Could you check a few things on this model? Use its own coordinates, in mm. Give positions to 0.01 mm unless a question says otherwise; leave off trailing zeros. Order: outer loops, then holes, each group sorted by start corner. A loop starts at its lowest first (then second) coordinate and runs counter-clockwise, first axis right, second up. Notation, with made-up numbers: (-15, -9.75) -> (19, -9.75) arc R17 ccw to (19, 9.25) -> close; hole circle Ø7 at (9.5, 7.5). An arc over 180 degrees is marked (long way). One line per item, written item: value.
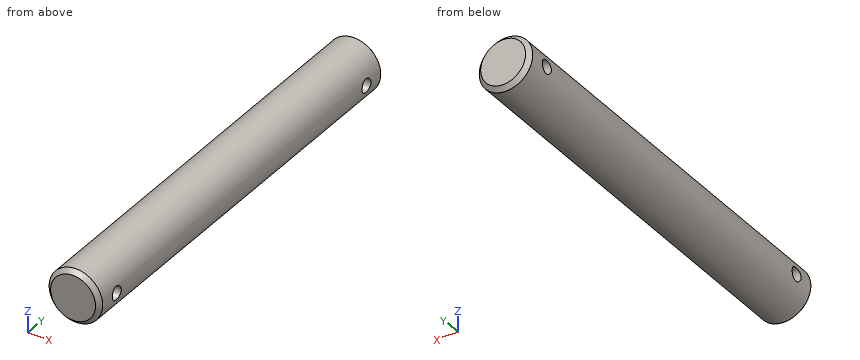
```python
from build123d import *

# Parameters (mm, degrees)
F0_R     = 12.5
F1_DEPTH = 200
F2_R     = 3.15
F3_DEPTH = 65
F4_SIZE  = 2


with BuildPart() as f1:
    # F0 (on Front) → F1 (new body)
    with BuildSketch(Plane.XZ):
        Circle(F0_R)
    extrude(amount=F1_DEPTH)

    # F2 (on Right) → F3 (cut, symmetric)
    with BuildSketch(Plane.YZ):
        with Locations((-12, 0)):
            Circle(F2_R)
        with Locations((-188, 0)):
            Circle(F2_R)
    extrude(amount=F3_DEPTH, both=True, mode=Mode.SUBTRACT)

    # F4
    f4_edges = [f1.edges().sort_by_distance(p)[0] for p in [
        (-12.5, 0, 0),
        (-12.5, -200, 0),
    ]]
    chamfer(f4_edges, length=F4_SIZE)


solid = f1.part
```
1) Suppose I cut it at C-C, the plane y = -90.5. Write out the boundary of the cut face in (x, z).
Answer below:
outline: circle Ø25 at (0, 0)
2) For P1, Ø10, axis at x = 5, y = -38, coming from the +Z side; P2, Ø4, axis at y = -46.5, z = -5.5, coming from the +X side; P3, Ø4, axis at y = -88.5, z = -8, coming from the -X side, each with a flat end and sliding along its axis, tell me the tip position at first contact or that it passes through.
Answer below:
P1: stops at z = 12.5
P2: stops at x = 12
P3: stops at x = -10.97
3) If I drill on line 1 along Y through (x, z) = (-4.25, 0); line 2 along Z through (x, y) = (6.75, -188); line 3 along Z through (x, y) = (0.5, -67), over which ranges is the centre line in solid material (lowest first)?
Answer below:
line 1: y = -200 to -191.15, -184.85 to -15.15, -8.85 to 0
line 2: z = -10.52 to -3.15, 3.15 to 10.52
line 3: z = -12.49 to 12.49
4) Suppose I cut it at B-B, the plane x = 6.75. State how many separate pieces and enclosed holes the cut face has, then the cut area to 3 significant figures.
Answer below:
separate pieces: 1
enclosed holes: 2
area: 4,140 mm2
5) Suppose I cut it at A-A, the plane y = -188. Write out the boundary of the cut face in (x, z).
Answer below:
outline: (-12.1, -3.15) arc R12.5 ccw to (12.1, -3.15) -> close; (-12.1, 3.15) -> (12.1, 3.15) arc R12.5 ccw to start
